Read the model definition and answer for the solid it produces. Units are mm, in the model's axes. Face numbers are marked on the shaded views. A direction names the side the tool comes from. Round coordinates to 2 decimals unless told otherwise and drop trailing zeros. Loops run counter-clockwise (first coordinate to the right, second up) from the corner with the lowest first, then second, coordinate; pieces in that order, holes last. Notation, with made-up numbers: M 40,23.5 L 99,23.5 A24 cw 99,62.5 Z; hole C -17.5,77 d7. An arc over 180 degrees is marked long. Write each question's results on one line, items separated by ' | '.
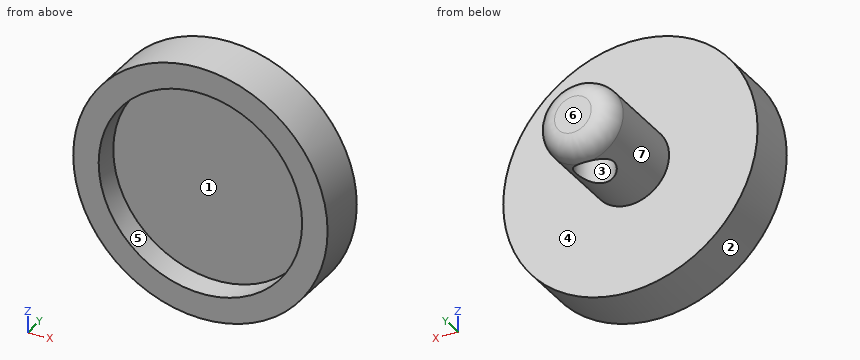
from build123d import *

# Parameters (mm, degrees)
SKETCH3_R          = 2.38125
CUT_EXTRUDE1_DEPTH = 19.045054718


with BuildPart() as part:
    # Sketch1 → Revolve1 (revolve)
    with BuildSketch(Plane.XY):
        with BuildLine():
            Line((0, 0), (2.286, 0))
            ThreePointArc((2.286, 0), (4.082051224, -0.743948776), (4.826, -2.54))
            Line((4.826, -2.54), (4.826, -12.5095))
            Line((4.826, -12.5095), (15.875, -12.5095))
            Line((15.875, -12.5095), (15.875, -18.8595))
            Line((15.875, -18.8595), (12.7, -18.8595))
            Line((12.7, -18.8595), (12.7, -15.6845))
            Line((12.7, -15.6845), (0, -15.6845))
            Line((0, -15.6845), (0, 0))
        make_face()
    revolve(axis=Axis((0, 0, 0), (0, -1, 0)))

    # Sketch3 → Cut-Extrude1 (cut)
    with BuildSketch(Plane.XY.offset(4.826)):
        with Locations((0, -4.7625)):
            Circle(SKETCH3_R)
    extrude(amount=-CUT_EXTRUDE1_DEPTH, mode=Mode.SUBTRACT)


solid = part.part
Item 1: Flat-ended cylindrical pins translate along their axes: pin 1 (6 mm diameter, centred on x = 11.5, y = -16.5, fed in from +Z); pin 2 (5.5 mm diameter, centred on x = 0, y = -4.76, fed in from -Z); pin 3 (8 mm diameter, centred on x = -3, y = -6, fed in from +Z); pin 4 (8 mm diameter, centred on y = -5, z = -12, fed in from +X). Find the tip coordinate at first contact, or state that the pin passes through.
Outcome:
pin 1: stops at z = 13.41 | pin 2: stops at z = -4.83 | pin 3: stops at z = 4.83 | pin 4: passes through
Item 2: The part is cut by section B-B (z = -9). Determine the outline of the cut face in (x, y).
Outcome:
outline: M -13.08,-18.86 L -8.96,-18.86 L -8.96,-15.68 L 8.96,-15.68 L 8.96,-18.86 L 13.08,-18.86 L 13.08,-12.51 L -13.08,-12.51 Z
Item 3: The part is cut by section A-A (x = 8). Determine the outline of the cut face in (y, z), plus the area to 3 significant figures.
Outcome:
outline: M -18.86,-13.71 L -12.51,-13.71 L -12.51,13.71 L -18.86,13.71 L -18.86,9.86 L -15.68,9.86 L -15.68,-9.86 L -18.86,-9.86 Z | area: 112 mm2
Item 4: The mould has two halves that part along X. Classify the marked faces 1, 2, 3 and 4: pulls with the +X half, pulls with the -X half, needs draft (parallel to the pull), parting line crosses it, or undercut.
Outcome:
face 1: undercut | face 2: parting line crosses it | face 3: undercut | face 4: needs draft
Item 5: Straight lines are drawn through the part: line 1 (Z direction, x = 0, y = -16) (3 decimals); line 2 (Y direction, x = 4, z = 13); line 3 (Y direction, x = 0, z = 1.25). For each, find the intervals that lie inside material, in ascending order.
Outcome:
line 1: z = -15.875 to -12.7, 12.7 to 15.875 | line 2: y = -18.86 to -12.51 | line 3: y = -15.68 to -7.14, -2.38 to 0
Item 6: The part is cut by section D-D (y = -14). Determine the outline of the cut face in (x, z) (3 decimals), plus the area to 3 significant figures.
Outcome:
outline: C 0,0 d31.75 | area: 792 mm2
Item 7: For the marked faces 5, 6 and 7, determine the directions among +Z, -Z, +X, -X, +Y, -Y from which every point of the face is accessible in a straight line to the end or side of a thin tool.
Outcome:
face 5: -Y | face 6: +Z, -Z, +X, -X, +Y | face 7: +Y
Item 8: The part is cut by section C-C (y = -3.5). Determine the outline of the cut face in (x, z), plus the area to 3 significant figures.
Outcome:
outline: M -2.02,-4.38 L -2.02,4.38 A4.83 ccw Z; M 2.02,-4.38 A4.83 ccw 2.02,4.38 Z | area: 35.4 mm2
